```python
from build123d import *

# Parameters (mm, degrees)
SKETCH1_W           = 10
SKETCH1_H           = 10
BOSS_EXTRUDE1_DEPTH = 10
SKETCH1_4_R         = 7.4
BOSS_EXTRUDE2_DEPTH = 5
FILLET1_R           = 1
BOSS_EXTRUDE3_START = 5
SKETCH2_R           = 12
BOSS_EXTRUDE3_DEPTH = 2


with BuildPart() as part:
    # Sketch1 → Boss-Extrude1 (new body)
    with BuildSketch(Plane.XY):
        Rectangle(SKETCH1_W, SKETCH1_H)
    extrude(amount=-BOSS_EXTRUDE1_DEPTH)

    # Sketch1<4> → Boss-Extrude2 (add)
    with BuildSketch(Plane.XY):
        Circle(SKETCH1_4_R)
    extrude(amount=BOSS_EXTRUDE2_DEPTH)

    # Fillet1
    fillet1_edges = [part.edges().sort_by_distance(p)[0] for p in [
        (-5, -5, -5),
        (-5, 5, -5),
        (5, 5, -5),
        (5, -5, -5),
    ]]
    fillet(fillet1_edges, radius=FILLET1_R)

    # Sketch2 → Boss-Extrude3 (add)
    with BuildSketch(Plane.XY.offset(BOSS_EXTRUDE3_START)):
        Circle(SKETCH2_R)
    extrude(amount=BOSS_EXTRUDE3_DEPTH)


solid = part.part
```
Geometry check sheet. Reference: the model listing, model coordinates, mm. A direction names the side the tool comes from. Give positions to 0.01 mm unless a question says otherwise; leave off trailing zeros. Order: outer loops, then holes, each group sorted by start corner. A loop starts at its lowest first (then second) coordinate and runs counter-clockwise, first axis right, second up.
1. Gauge pin test, flat ends, axial feed: pin 1 Ø9 at (x, z) = (1, -2.5) entering from +Y; pin 2 Ø12 at (x, y) = (2, -8) entering from -Z; pin 3 Ø4 at (y, z) = (-9.5, -3) entering from -X; pin 4 Ø8 at (x, z) = (6.5, -7) entering from +Y. Record the tip position at first contact, or that the pin passes through.
2. Section check A-A, the plane y = 0. Enter the section's corners in (x, z), and give its area (3 significant figures).
3. Section check C-C, the plane z = -6. Enter the section's corners in (x, y).
4. Access from +Z, -Z, +X, -X, +Y, -Y to the whole of each face (thin tool, end or side, straight path). Record for faces 1 (the face through (4.699, -4.715, -5.07)), 2 (the face through (0, 5, -5)), 3 (the face through (-5, 0, -5)), 4 (the face through (-4.699, 4.715, -5.07)), 5 (the face through (5, 6, 5)).
5. Section check D-D, the plane z = 3.25. Enter the section's corners in (x, y), and give its area (3 significant figures).
6. Thickness scan on L1, parallel to Z at x = -10.25, y = -3.5; L2, parallel to Y at x = -0.75, z = -7.25; L3, parallel to Z at x = 5.25, y = 3.25. Record the ranges inside material, lowest first.
Values follow:
1. pin 1: stops at y = 7.4
1. pin 2: stops at z = -10
1. pin 3: passes through
1. pin 4: stops at y = 5
2. outline: (-12, 5) - (-7.4, 5) - (-7.4, 0) - (-5, 0) - (-5, -10) - (5, -10) - (5, 0) - (7.4, 0) - (7.4, 5) - (12, 5) - (12, 7) - (-12, 7) - close
2. area: 222 mm2
3. outline: (-5, -4) arc R1 ccw to (-4, -5) - (4, -5) arc R1 ccw to (5, -4) - (5, 4) arc R1 ccw to (4, 5) - (-4, 5) arc R1 ccw to (-5, 4) - close
4. face 1: -Z, +X, -Y
4. face 2: -Z, +X, -X, +Y
4. face 3: -Z, -X, +Y, -Y
4. face 4: -Z, -X, +Y
4. face 5: -Z
5. outline: circle Ø14.8 at (0, 0)
5. area: 172 mm2
6. L1: z = 5 to 7
6. L2: y = -5 to 5
6. L3: z = 0 to 7
